```python
from build123d import *

# Parameters (mm, degrees)
TABAN_FLAN_2_DEPTH    = 60
RADYUS1_R             = 20
RADYUS2_R             = 2
IZIM10_R              = 17.5
KES_EKSTR_ZYON1_DEPTH = 30


# Sheet-metal steps are written as plain solids
with BuildPart() as part:
    # Çizim1 → Taban-Flanş2 (new body)
    with BuildSketch(Plane.XY):
        with BuildLine():
            Line((0, 0), (0, -85))
            ThreePointArc((0, -85), (4.393398282, -95.606601718), (15, -100))
            Line((15, -100), (40, -100))
            Line((40, -100), (40, -90))
            Line((40, -90), (15, -90))
            ThreePointArc((15, -90), (11.464466094, -88.535533906), (10, -85))
            Line((10, -85), (10, 0))
            Line((10, 0), (0, 0))
        make_face()
    extrude(amount=TABAN_FLAN_2_DEPTH)

    # Radyus1
    radyus1_edges = [part.edges().sort_by_distance(p)[0] for p in [
        (5, 0, 0),
        (5, 0, 60),
    ]]
    fillet(radyus1_edges, radius=RADYUS1_R)

    # Radyus2
    radyus2_edges = [part.edges().sort_by_distance(p)[0] for p in [
        (40, -95, 0),
        (40, -95, 60),
    ]]
    fillet(radyus2_edges, radius=RADYUS2_R)

    # Çizim10 → Kes-Ekstrüzyon1 (cut)
    with BuildSketch(Plane.ZY):
        with Locations(Location((30, -30, 0), (0, 0, 270))):
            Circle(IZIM10_R)
    extrude(amount=-KES_EKSTR_ZYON1_DEPTH, mode=Mode.SUBTRACT)


solid = part.part
```
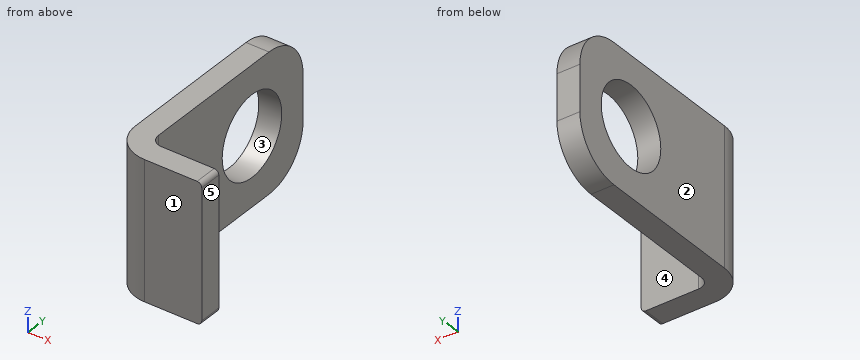
Design review of the part built by this model. Coordinates are the model's own, in mm. Face numbers are marked on the shaded views. A direction names the side the tool comes from. Coordinates: 2 decimals unless noted, no trailing zeros. Order: outer loops, then holes, each group sorted by start corner. A loop starts at its lowest first (then second) coordinate and runs counter-clockwise, first axis right, second up. Notation, with made-up numbers: (-29.75, -38) - (-14.75, -38) arc R25 ccw to (-14.75, -18) - close; hole circle Ø3 at (-33.75, 38). An arc over 180 degrees is marked (long way). Answer in a Markdown table with one row per item.
(1) Consider section D-D on y = -73. State the section outline as (x, z) points.
Checked values:
| item | result |
|---|---|
| outline | (0, 0) - (10, 0) - (10, 60) - (0, 60) - close |
(2) Clearance check with flat-ended pins moving along their axes: pin 1 (3 mm diameter, centred on y = -11, z = 41, fed in from +X); pin 2 (6 mm diameter, centred on x = 15, z = 26.5, fed in from +Y); pin 3 (12.5 mm diameter, centred on x = 33.5, z = 20.5, fed in from +Y). State where each tip first meets the part, or that it passes through.
Checked values:
| item | result |
|---|---|
| pin 1 | x = 10 |
| pin 2 | y = -89 |
| pin 3 | y = -90 |
(3) Consider section B-B on y = -42. State the section outline as (x, z) points.
Checked values:
| item | result |
|---|---|
| outline | (0, 0) - (10, 0) - (10, 17.26) - (0, 17.26) - close; (0, 42.74) - (10, 42.74) - (10, 60) - (0, 60) - close |
(4) Consider section C-C on x = 8. State the section outline as (y, z) points.
Checked values:
| item | result |
|---|---|
| outline | (-98.27, 0) - (-20, 0) arc R20 ccw to (0, 20) - (0, 40) arc R20 ccw to (-20, 60) - (-98.27, 60) - close; hole circle Ø35 at (-30, 30) |
(5) Wall thickness on line 1 along Z through (x, y) = (5.25, -30); line 2 along Y through (x, z) = (36, 18.5); line 3 along X through (y, z) = (-29, 56): over which ranges is each line inside the solid? List them lowest first. Write a range as from..to.
Checked values:
| item | result |
|---|---|
| line 1 | 0..12.5, 47.5..60 |
| line 2 | -100..-90 |
| line 3 | 0..10 |
(6) For the marked faces 4 and 5, list the 3-axis set-ups (+Z, -Z, +X, -X, +Y, -Y) from which the entire face can be reached by the end or side of a thin tool; tool diameter is ignored.
Checked values:
| item | result |
|---|---|
| face 4 | +Z, -Z, +X, +Y |
| face 5 | +Z, -Z, +X, +Y, -Y |
(7) The part is to be moulded in two halves that separate along Y. For the marked faces 1, 2 and 3, say which applies: released by +Y, released by -Y, zero draft, split by the parting line, or undercut.
Checked values:
| item | result |
|---|---|
| face 1 | released by -Y |
| face 2 | zero draft |
| face 3 | undercut |
(8) Consider section A-A on z = 30. State the section outline as (x, y) points.
Checked values:
| item | result |
|---|---|
| outline | (0, -85) arc R15 ccw to (15, -100) - (40, -100) - (40, -90) - (15, -90) arc R5 cw to (10, -85) - (10, -47.5) - (0, -47.5) - close; (0, -12.5) - (10, -12.5) - (10, 0) - (0, 0) - close |
